```python
from build123d import *

# Parameters (mm, degrees)
CUT_EXTRUDE_3_DEPTH    = 11.5
HOLE_WIZARD_M3_1_D     = 2.5
HOLE_WIZARD_M3_1_DEPTH = 5.5
HOLE_WIZARD_M3_1_TIP   = 0.751075774
SKETCH_12_R            = 1.5
CUT_EXTRUDE_4_DEPTH    = 11.5
HOLE_WIZARD_M3_2_D     = 2.5
HOLE_WIZARD_M3_2_DEPTH = 4
HOLE_WIZARD_M3_2_TIP   = 0.751075774
EXTRUDE_START          = 0.5
EXTRUDE_1_DEPTH        = 0.5


with BuildPart() as part:
    # 草图1 → 旋转1 (revolve)
    with BuildSketch(Plane(origin=(0, 0, 0), x_dir=(1, 0, 0), z_dir=(0, 1, 0))):
        Polygon((0, 0), (-29, 0), (-29, 5.7), (-31.6, 5.7), (-31.6, 9.2), (-46, 9.2), (-46, 12.2), (0, 12.2), align=None)
    revolve(axis=Axis((-46, 0, -12.2), (1, 0, 0)))

    # 草图9 → 切除-拉伸3 (cut)
    with BuildSketch(Plane.ZY.offset(46)):
        with BuildLine():
            Line((-12.2, 2.5), (-10.541687605, 2.5))
            ThreePointArc((-10.541687605, 2.5), (-12.2, 3), (-13.858312395, 2.5))
            Line((-13.858312395, 2.5), (-12.2, 2.5))
        make_face()
    extrude(amount=-CUT_EXTRUDE_3_DEPTH, mode=Mode.SUBTRACT)

    # M3 螺纹孔1
    with Locations(Plane.ZY.offset(46)):
        with Locations((-12.2, 0)):
            Hole(HOLE_WIZARD_M3_1_D / 2, depth=HOLE_WIZARD_M3_1_DEPTH)
            with Locations((0, 0, -(HOLE_WIZARD_M3_1_DEPTH + HOLE_WIZARD_M3_1_TIP / 2))):  # 118° drill point
                Cone(0, HOLE_WIZARD_M3_1_D / 2, HOLE_WIZARD_M3_1_TIP, mode=Mode.SUBTRACT)

    # 草图12 → 切除-拉伸4 (cut)
    with BuildSketch(Plane(origin=(0, 2.5, 0), x_dir=(1, 0, 0), z_dir=(0, 1, 0))):
        with Locations(Location((-37, 12.2, 0), (0, 0, 270))):
            Circle(SKETCH_12_R)
    extrude(amount=-CUT_EXTRUDE_4_DEPTH, mode=Mode.SUBTRACT)

    # M3 螺纹孔2
    with Locations(Plane.ZY.offset(29)):
        with Locations((-12.2, 9.5), (-20.427241336, -4.75), (-3.972758664, -4.75)):
            Hole(HOLE_WIZARD_M3_2_D / 2, depth=HOLE_WIZARD_M3_2_DEPTH)
            with Locations((0, 0, -(HOLE_WIZARD_M3_2_DEPTH + HOLE_WIZARD_M3_2_TIP / 2))):  # 118° drill point
                Cone(0, HOLE_WIZARD_M3_2_D / 2, HOLE_WIZARD_M3_2_TIP, mode=Mode.SUBTRACT)

    # 草图16 → 凸台-拉伸1 (add)
    with BuildSketch(Plane.ZY.offset(31.6).offset(EXTRUDE_START)):
        with BuildLine():
            Line((-9.601923789, -1.5), (-12.2, -6))
            ThreePointArc((-12.2, -6), (-8.525765386, 4.74341649), (-18.009475019, -1.5))
            Line((-18.009475019, -1.5), (-14.69206472, 1.670213589))
            ThreePointArc((-14.69206472, 1.670213589), (-10.614007201, 2.546493048), (-9.601923789, -1.5))
        make_face()
    extrude(amount=-EXTRUDE_1_DEPTH)


solid = part.part
```
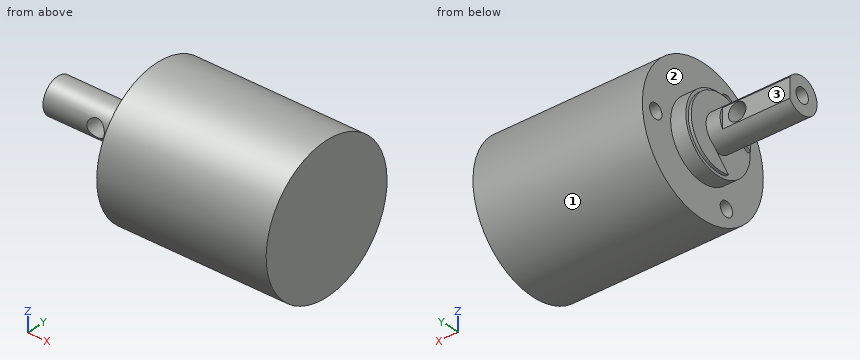
The model under review builds one solid part; all positions refer to its coordinate system, in mm. Face numbers are marked on the shaded views. A direction names the side the tool comes from. Round coordinates to 2 decimals unless told otherwise and drop trailing zeros. Order: outer loops, then holes, each group sorted by start corner. A loop starts at its lowest first (then second) coordinate and runs counter-clockwise, first axis right, second up.
(1) Wall thickness on L1, parallel to Y at x = -42.5, z = -12.2; L2, parallel to Z at x = -42.25, y = 0; L3, parallel to Z at x = -26.3, y = -4.75: over which ranges is each line inside the solid? List them lowest first.
Working result:
L1: y = -3 to -1.25, 1.25 to 2.5
L2: z = -15.2 to -13.45, -10.95 to -9.2
L3: z = -23.44 to -21.68, -19.18 to -5.22, -2.72 to -0.96
(2) Take a section at C-C, the plane y = 5.5. State the section outline as (x, z) points, plus the area to 3 significant figures.
Working result:
outline: (-32.1, -14.6) - (-31.6, -14.6) - (-31.6, -15.66) - (-29, -15.66) - (-29, -23.09) - (0, -23.09) - (0, -1.31) - (-29, -1.31) - (-29, -8.74) - (-31.6, -8.74) - (-31.6, -9.8) - (-32.1, -9.8) - close
area: 652 mm2
(3) Take a section at A-A, the plane x = -37. State the section outline as (y, z) points, plus the area to 3 significant figures.
Working result:
outline: (-2.6, -13.7) arc R3 ccw to (2.5, -13.86) - (2.5, -13.7) - close; (-2.6, -10.7) - (2.5, -10.7) - (2.5, -10.54) arc R3 ccw to start
area: 11.0 mm2
(4) Tool access review of the marked faces 1, 2 and 3: name each direction out of +Z, -Z, +X, -X, +Y, -Y from which nothing blocks a thin tool from reaching the whole face with its end or side.
Working result:
face 1: +X, -X
face 2: -X
face 3: +Z, -Z, -X, +Y
(5) For P1, Ø1, axis at y = -6, z = -8.5, coming from the -X side; P2, Ø2, axis at x = -19, z = -6.5, coming from the +Y side; P3, Ø5, axis at x = -11, z = -7.5, coming from the -Y side, all flat-tipped, find the tip position at first contact; note any pin that passes through.
Working result:
P1: stops at x = -29
P2: stops at y = 11.26
P3: stops at y = -12
(6) Take a section at B-B, the plane y = -2. State the section outline as (x, z) points, plus the area to 3 significant figures.
Working result:
outline: (-46, -14.44) - (-31.6, -14.44) - (-31.6, -18.38) - (-29, -18.38) - (-29, -24.23) - (0, -24.23) - (0, -0.17) - (-29, -0.17) - (-29, -6.02) - (-31.6, -6.02) - (-31.6, -6.54) - (-32.1, -6.54) - (-32.1, -9.89) - (-31.6, -9.89) - (-31.6, -9.96) - (-46, -9.96) - close; hole circle Ø3 at (-37, -12.2)
area: 789 mm2
(7) Take a section at D-D, the plane z = -1.5. State the section outline as (x, y) points, plus the area to 3 significant figures.
Working result:
outline: (-29, -5.86) - (0, -5.86) - (0, 5.86) - (-29, 5.86) - close
area: 340 mm2
